Here's how the part is built. I have some questions about the finished solid (model axes, mm). A direction names the side the tool comes from. Give positions to 0.01 mm unless a question says otherwise; leave off trailing zeros. Loops run counter-clockwise (first coordinate to the right, second up) from the corner with the lowest first, then second, coordinate; pieces in that order, holes last. Notation, with made-up numbers: (59, 14.25) - (79, 14.25) arc R15 ccw to (79, 34.25) - close; hole circle Ø11 at (19.25, -11). An arc over 180 degrees is marked (long way). Return JSON: item names as keys, results as strings. Group by question number.
(1) If we mould it in two halves opening along X, with no side actions, what happens to faces 1 (the flat face through (29.658, 92, 1)), 2 (the flat face through (-24.4, 89.67, 7.58)), 3 (the cylindrical face through (-17.518, 91.745, 6.409))? For each: released by +X, released by -X, zero draft, split by the parting line, or undercut.
(2) If we section it at C-C (z = 9): Please give me the cut outline in (x, y), then the cut area to 3 significant figures.
(3) If we section it at B-B (x = -8.5): Please give me the cut outline in (y, z), then the cut area to 3 significant figures.
(4) For P1, Ø6, axis at x = -18, z = 8.5, coming from the -Y side; P2, Ø3.5, axis at x = 3, z = 5.5, coming from the +Y side; P3, Ø8, axis at x = 20.5, y = 93, coming from the -Z side; P4, Ø6, axis at x = 13.5, z = 9.5, coming from the -Y side, each with a flat end and sliding along its axis, tell me the tip position at first contact or that it passes through.
(5) If we section it at D-D (z = 1.5): Please give me the cut outline in (x, y).
(6) If we section it at A-A (z = 4.25): Please give me the cut outline in (x, y), then the cut area to 3 significant figures.
(7) I need wall thicknesses on probe 1 along Z at (x, y) = (21, 97.25); probe 2 along Y at (x, z) = (6, 7.5); probe 3 along Z at (x, y) = (-23.5, 90.5). Which ranges of each line are inside material? Lowest first, please. Write a range as [from, to].
(8) On a 3-axis mill with a long thin cutter (end or side, diameter ignored), from which of +Z, -Z, +X, -X, +Y, -Y can I reach the whole of each face in a straight line? I mean faces 4 (the flat face through (0, 94.2, 8)), 5 (the flat face through (0, 94, 0)), 6 (the flat face through (24.33, 89.76, 7.58)), 7 (the flat face through (0, 91.9, 6)). Say none if no direction works.
```python
from build123d import *

# Parameters (mm, degrees)
EXTRUDE_5_DEPTH          = 30
EXTRUDE_6_DEPTH          = 2
CUT_EXTRUDE_7_DEPTH      = 10
CUT_EXTRUDE_7_DEPTH_BACK = 10
EXTRUDE_8_DEPTH          = 13
SKETCH_14_R              = 1.6
CUT_EXTRUDE_8_DEPTH      = 10
SKETCH_21_R              = 3.5
CUT_EXTRUDE_10_DEPTH     = 10
FILLET_3_R               = 3
CUT_EXTRUDE_9_DEPTH      = 11
EXTRUDE_7_DEPTH          = 2


with BuildPart() as part:
    # 草图1<3> → 凸台-拉伸5 (new body)
    with BuildSketch(Plane.XY):
        with BuildLine():
            Line((-20.937049459, 94.3), (-26.657578158, 87.182553786))
            Line((-26.657578158, 87.182553786), (-24.786904599, 85.67903111))
            Line((-24.786904599, 85.67903111), (-22.188666929, 88.911742253))
            ThreePointArc((-22.188666929, 88.911742253), (-19.410403975, 91.114358531), (-15.9530884, 91.9))
            Line((-15.9530884, 91.9), (15.9530884, 91.9))
            ThreePointArc((15.9530884, 91.9), (19.410403975, 91.114358531), (22.188666929, 88.911742253))
            Line((22.188666929, 88.911742253), (24.786904599, 85.67903111))
            Line((24.786904599, 85.67903111), (26.657578158, 87.182553786))
            Line((26.657578158, 87.182553786), (20.937049459, 94.3))
            Line((20.937049459, 94.3), (-20.937049459, 94.3))
        make_face()
    extrude(amount=EXTRUDE_5_DEPTH)

    # 草图12 → 凸台-拉伸6 (add)
    with BuildSketch(Plane(origin=(0, 0, 0), x_dir=(-1, 0, 0), z_dir=(0, 0, -1))):
        Polygon((20.937049459, 94.3), (26.657578158, 87.182553786), (26.657578158, 95.163810199), (23.333184583, 99.3), (-23.333184583, 99.3), (-26.657578158, 95.163810199), (-26.657578158, 87.182553786), (-20.937049459, 94.3), align=None)
    extrude(amount=-EXTRUDE_6_DEPTH)

    # 草图13 → 切除-拉伸7 (cut, two sides: drawn at the far end of the back side and taken through both)
    with BuildSketch(Plane.XZ.offset(-91.9).offset(-CUT_EXTRUDE_7_DEPTH_BACK)):
        Polygon((-15.9530884, 13), (15.9530884, 13), (26.657578158, 13), (26.657578158, 30), (-26.657578158, 30), (-26.657578158, 13), align=None)
    extrude(amount=CUT_EXTRUDE_7_DEPTH + CUT_EXTRUDE_7_DEPTH_BACK, mode=Mode.SUBTRACT)

    # 草图20 → 凸台-拉伸8 (add)
    with BuildSketch(Plane.XY.offset(13)):
        Polygon((-24.786904599, 85.67903111), (-19.762367643, 91.930528728), (-18.982920327, 91.304060946), (-24.007457283, 85.052563329), align=None)
    extrude_8 = extrude(amount=-EXTRUDE_8_DEPTH)

    # 草图14 → 切除-拉伸8 (cut, symmetric)
    with BuildSketch(Plane(origin=(-56.116495667, 45.102697556, 0), x_dir=(0, 0, -1), z_dir=(0.7794473160570586, -0.6264677816866944, 0))):
        with Locations(Location((-8.5, 56.385494975, 0), (0, 0, 90))):
            Circle(SKETCH_14_R)
    cut_extrude_8 = extrude(amount=CUT_EXTRUDE_8_DEPTH, both=True, mode=Mode.SUBTRACT)

    # 草图21 → 切除-拉伸10 (cut)
    with BuildSketch(Plane(origin=(-56.116495667, 45.102697556, 0), x_dir=(0, 0, -1), z_dir=(0.7794473160570586, -0.6264677816866944, 0))):
        with Locations((-8.5, 56.385494975)):
            Circle(SKETCH_21_R)
    cut_extrude_10 = extrude(amount=CUT_EXTRUDE_10_DEPTH, mode=Mode.SUBTRACT)

    # 镜向2: 凸台-拉伸8, 切除-拉伸8, 切除-拉伸10 across plane
    add(extrude_8.mirror(Plane(origin=(0, 0, 0), x_dir=(0, 0, 1), z_dir=(1, 0, 0))))
    add(cut_extrude_8.mirror(Plane(origin=(0, 0, 0), x_dir=(0, 0, 1), z_dir=(1, 0, 0))), mode=Mode.SUBTRACT)
    add(cut_extrude_10.mirror(Plane(origin=(0, 0, 0), x_dir=(0, 0, 1), z_dir=(1, 0, 0))), mode=Mode.SUBTRACT)

    # 圆角3
    fillet_3_edges = [part.edges().sort_by_distance(p)[0] for p in [
        (-20.937049459, 94.3, 7.5),
        (20.937049459, 94.3, 7.5),
    ]]
    fillet(fillet_3_edges, radius=FILLET_3_R)

    # 草图15 → 切除-拉伸9 (cut)
    with BuildSketch(Plane.XY.offset(13)):
        with BuildLine():
            ThreePointArc((21.837710333, 93.179403345), (21.455277133, 93.574735362), (21.007094419, 93.89360024))
            Line((21.007094419, 93.89360024), (26.501688695, 87.05726023))
            Line((26.501688695, 87.05726023), (26.657578158, 87.182553786))
            Line((26.657578158, 87.182553786), (21.837710333, 93.179403345))
        make_face()
        with BuildLine():
            Line((-26.657578158, 87.182553786), (-26.501688695, 87.05726023))
            Line((-26.501688695, 87.05726023), (-21.007094419, 93.89360024))
            ThreePointArc((-21.007094419, 93.89360024), (-21.455277133, 93.574735362), (-21.837710333, 93.179403345))
            Line((-21.837710333, 93.179403345), (-26.657578158, 87.182553786))
        make_face()
        with BuildLine():
            ThreePointArc((-19.499368384, 94.3), (-19.886666719, 94.274894956), (-20.267482959, 94.2))
            Line((-20.267482959, 94.2), (20.267482959, 94.2))
            ThreePointArc((20.267482959, 94.2), (19.886666719, 94.274894956), (19.499368384, 94.3))
            Line((19.499368384, 94.3), (-19.499368384, 94.3))
        make_face()
    extrude(amount=-CUT_EXTRUDE_9_DEPTH, mode=Mode.SUBTRACT)

    # 草图17 → 凸台-拉伸7 (add)
    with BuildSketch(Plane.XY.offset(2)):
        Polygon((-29.657578158, 89.593753756), (-26.657578158, 87.182553786), (-26.657578158, 95.163810199), (-23.333184583, 99.3), (-25.89910528, 99.3), (-29.657578158, 94.62373143), align=None)
        Polygon((23.333184583, 99.3), (26.657578158, 95.163810199), (26.657578158, 87.182553786), (29.657578158, 89.593753756), (29.657578158, 94.62373143), (25.89910528, 99.3), align=None)
    extrude(amount=-EXTRUDE_7_DEPTH)


solid = part.part
```
Values:
{
 "1": {"face 1": "released by +X", "face 2": "released by -X", "face 3": "undercut"},
 "2": {"outline": "(-26.5, 87.06) - (-24.01, 85.05) - (-21.74, 87.87) - (-24.24, 89.87) - close; (-22.33, 92.24) - (-19.84, 90.24) - (-18.62, 91.75) - (-18.35, 91.53) arc R8 cw to (-15.95, 91.9) - (15.95, 91.9) arc R8 cw to (18.35, 91.53) - (18.62, 91.75) - (19.84, 90.24) - (22.33, 92.24) - (21.01, 93.89) arc R3 ccw to (20.27, 94.2) - (-20.27, 94.2) arc R3 ccw to (-21.01, 93.89) - close; (21.74, 87.87) - (24.01, 85.05) - (26.5, 87.06) - (24.24, 89.87) - close", "area": "129 mm2"},
 "3": {"outline": "(91.9, 0) - (99.3, 0) - (99.3, 2) - (94.2, 2) - (94.2, 13) - (91.9, 13) - close", "area": "40.1 mm2"},
 "4": {"P1": "y = 89.34", "P2": "y = 94.2", "P3": "z = 0", "P4": "y = 91.88"},
 "5": {"outline": "(-29.66, 89.59) - (-24.01, 85.05) - (-18.98, 91.3) arc R8 cw to (-15.95, 91.9) - (15.95, 91.9) arc R8 cw to (18.98, 91.3) - (24.01, 85.05) - (29.66, 89.59) - (29.66, 94.62) - (25.9, 99.3) - (-25.9, 99.3) - (-29.66, 94.62) - close"},
 "6": {"outline": "(-26.5, 87.06) - (-24.01, 85.05) - (-18.98, 91.3) arc R8 cw to (-15.95, 91.9) - (15.95, 91.9) arc R8 cw to (18.98, 91.3) - (24.01, 85.05) - (26.5, 87.06) - (21.01, 93.89) arc R3 ccw to (20.27, 94.2) - (-20.27, 94.2) arc R3 ccw to (-21.01, 93.89) - close", "area": "149 mm2"},
 "7": {"probe 1": "[0, 2]", "probe 2": "[91.9, 94.2]", "probe 3": "[0, 7], [10, 13]"},
 "8": {"face 4": "+Z, +X, -X, +Y", "face 5": "-Z, +X, -X, +Y, -Y", "face 6": "+Z, +X, +Y", "face 7": "+Z, -Z, -Y"}
}
